from build123d import *

# Parameters (mm, degrees)
SKETCH_1_W               = 45
SKETCH_1_H               = 45
EXTRUDE_1_DEPTH          = 15
SKETCH_2_R               = 19
CUT_EXTRUDE_1_DEPTH      = 36.178118199
SKETCH_5_W               = 15
SKETCH_5_H               = 15
EXTRUDE_2_DEPTH          = 12
SKETCH_6_R               = 3
CUT_EXTRUDE_4_DEPTH      = 35
SKETCH_7_R               = 1.5
CUT_EXTRUDE_5_DEPTH      = 44.834917702
CUT_EXTRUDE_6_DEPTH      = 6
CUT_EXTRUDE_6_DEPTH_BACK = 6
SKETCH_9_R               = 4.25
CUT_EXTRUDE_7_DEPTH      = 12
CHAMFER_1_SIZE           = 2
CHAMFER_2_SIZE           = 1
CHAMFER_3_SIZE           = 1
CHAMFER_4_SIZE           = 1


# Some blends are built 0.0001 mm under size
with BuildPart() as part:
    # 草图1 → 凸台-拉伸1 (new body)
    with BuildSketch(Plane(origin=(0, 0, 0), x_dir=(1, 0, 0), z_dir=(0, 1, 0))):
        Rectangle(SKETCH_1_W, SKETCH_1_H)
    extrude(amount=EXTRUDE_1_DEPTH)

    # 草图2 → 切除-拉伸1 (cut, through all)
    with BuildSketch(Plane(origin=(0, 15, 0), x_dir=(1, 0, 0), z_dir=(0, 1, 0))):
        with Locations(Location((0, 0, 0), (0, 0, 270))):
            Circle(SKETCH_2_R)
    extrude(amount=-CUT_EXTRUDE_1_DEPTH, mode=Mode.SUBTRACT)

    # 草图5 → 凸台-拉伸2 (add)
    with BuildSketch(Plane(origin=(0, 0, -22.5), x_dir=(-1, 0, 0), z_dir=(0, 0, -1))):
        with Locations((14, 7.5)):
            Rectangle(SKETCH_5_W, SKETCH_5_H)
        with Locations((-14, 7.5)):
            Rectangle(SKETCH_5_W, SKETCH_5_H)
    extrude(amount=EXTRUDE_2_DEPTH)

    # 草图6 → 切除-拉伸4 (cut)
    with BuildSketch(Plane(origin=(0, 0, -34.5), x_dir=(-1, 0, 0), z_dir=(0, 0, -1))):
        with Locations((-14, 7.5)):
            Circle(SKETCH_6_R)
        with Locations((14, 7.5)):
            Circle(SKETCH_6_R)
    extrude(amount=-CUT_EXTRUDE_4_DEPTH, mode=Mode.SUBTRACT)

    # 草图7 → 切除-拉伸5 (cut, through all)
    with BuildSketch(Plane(origin=(0, 15, 0), x_dir=(1, 0, 0), z_dir=(0, 1, 0))):
        with Locations(Location((-19.5, 19.5, 0), (0, 0, 270))):
            Circle(SKETCH_7_R)
        with Locations(Location((19.5, 19.5, 0), (0, 0, 90))):
            Circle(SKETCH_7_R)
        with Locations(Location((19.5, -19.5, 0), (0, 0, 270))):
            Circle(SKETCH_7_R)
        with Locations(Location((-19.5, -19.5, 0), (0, 0, 90))):
            Circle(SKETCH_7_R)
    extrude(amount=-CUT_EXTRUDE_5_DEPTH, mode=Mode.SUBTRACT)

    # 草图8 → 切除-拉伸6 (cut, two sides: drawn at the far end of the back side and taken through both)
    with BuildSketch(Plane(origin=(0, 7.5, 0), x_dir=(-1, 0, 0), z_dir=(0, -1, 0)).offset(-CUT_EXTRUDE_6_DEPTH_BACK)):
        with BuildLine():
            Line((-8.874983497, 19.032463528), (-8.029746973, 17.219847954))
            ThreePointArc((-8.029746973, 17.219847954), (-15.073713466, 11.566467151), (-18.711347307, 3.299315376))
            Line((-18.711347307, 3.299315376), (-20.680962813, 3.646611731))
            ThreePointArc((-20.680962813, 3.646611731), (-16.660420146, 12.783990009), (-8.874983497, 19.032463528))
        make_face()
        with BuildLine():
            Line((20.680962813, 3.646611731), (18.711347307, 3.299315376))
            ThreePointArc((18.711347307, 3.299315376), (15.073713466, 11.566467151), (8.029746973, 17.219847954))
            Line((8.029746973, 17.219847954), (8.874983497, 19.032463528))
            ThreePointArc((8.874983497, 19.032463528), (16.660420146, 12.783990009), (20.680962813, 3.646611731))
        make_face()
    extrude(amount=CUT_EXTRUDE_6_DEPTH + CUT_EXTRUDE_6_DEPTH_BACK, mode=Mode.SUBTRACT)

    # 草图9 → 切除-拉伸7 (cut)
    with BuildSketch(Plane(origin=(0, 0, -34.5), x_dir=(-1, 0, 0), z_dir=(0, 0, -1))):
        with Locations((-14, 7.5)):
            Circle(SKETCH_9_R)
        with Locations((14, 7.5)):
            Circle(SKETCH_9_R)
    extrude(amount=-CUT_EXTRUDE_7_DEPTH, mode=Mode.SUBTRACT)

    # 倒角1
    # the kernel refuses this chamfer: 2 mm, written as the material it takes off along each edge
    with BuildSketch(Plane(origin=(-18.711347307, 1.5, -3.299315376), x_dir=(-0.11838916494267775, 0, 0.9929672731888879), z_dir=(0, 1, 0)), Plane(origin=(18.711347307, 13.5, -3.299315376), x_dir=(0.11838916494267755, 0, 0.9929672731888879), z_dir=(0, -1, 0))) as chamfer_1_piece_1:
        with BuildLine():
            Line((2.121782819, 0), (-CHAMFER_1_SIZE * 0.055836389964, -CHAMFER_1_SIZE * 0.998439931872))
            Line((-CHAMFER_1_SIZE * 0.055836389964, -CHAMFER_1_SIZE * 0.998439931872), (0, 0))
            ThreePointArc((0, 0), (1.090799435, -0.029617755), (2.121782819, 0))
        make_face()
    extrude(amount=12, mode=Mode.SUBTRACT)

    # 倒角2
    chamfer_2_edges = [part.edges().sort_by_distance(p)[0] for p in [
        (22.5, 7.5, 22.5),
        (-22.5, 7.5, 22.5),
        (-22.5, 7.5, -22.5),
        (22.5, 7.5, -22.5),
    ]]
    chamfer(chamfer_2_edges, length=CHAMFER_2_SIZE - 0.0001)  # a hair under: the kernel refuses the full size

    # 倒角3
    chamfer_3_edges = [part.edges().sort_by_distance(p)[0] for p in [
        (18.25, 7.5, -22.5),
        (-9.75, 7.5, -22.5),
    ]]
    chamfer(chamfer_3_edges, length=CHAMFER_3_SIZE)

    # 倒角4
    chamfer_4_edges = [part.edges().sort_by_distance(p)[0] for p in [
        (6.5, 7.5, -34.5),
        (14, 15, -34.5),
        (21.5, 7.5, -34.5),
        (14, 0, -34.5),
        (-21.5, 7.5, -34.5),
        (-14, 15, -34.5),
        (-6.5, 7.5, -34.5),
        (-14, 0, -34.5),
    ]]
    chamfer(chamfer_4_edges, length=CHAMFER_4_SIZE)


solid = part.part
Read the model definition and answer for the solid it produces. Units are mm, in the model's axes. A direction names the side the tool comes from. Coordinates: 2 decimals unless noted, no trailing zeros. Loops run counter-clockwise (first coordinate to the right, second up) from the corner with the lowest first, then second, coordinate; pieces in that order, holes last. Notation, with made-up numbers: (82.25, 73) -> (109.25, 73) arc R8 ccw to (109.25, 79) -> close; hole circle Ø1 at (79, 67). An arc over 180 degrees is marked (long way). Answer in a Markdown table with one row per item.
Item 1: Straight lines are drawn through the part: line 1 along X through (y, z) = (5, 19.5); line 2 along X through (y, z) = (8, -1); line 3 along X through (y, z) = (8, -19.5). For each, find the intervals that lie inside material, in ascending order. Write a range as [from, to].
Returned:
| item | result |
|---|---|
| line 1 | x = [-22.5, -21], [-18, 18], [21, 22.5] |
| line 2 | x = [-22.5, -18.97], [18.97, 22.5] |
| line 3 | x = [-22.5, -21], [-18, -16.96], [-11.04, 11.04], [16.96, 18], [21, 22.5] |
Item 2: For faces 4 (the cylindrical face through (17, 7.6, -18.6)), 5 (the flat face through (-16, 13.5, -11)), 6 (the flat face through (14, 12, -34.5)), 7 (the flat face through (-10, 15, -18)), 8 (the flat face through (0, 7, -22.5)), determine the directions among +Z, -Z, +X, -X, +Y, -Y from which every point of the face is accessible in a straight line to the end or side of a thin tool.
Returned:
| item | result |
|---|---|
| face 4 | -Z |
| face 5 | none |
| face 6 | -Z, +X, -X, +Y, -Y |
| face 7 | +Z, -Z, +X, -X, +Y |
| face 8 | -Z, +Y, -Y |
Item 3: A cutting plane is placed at A-A on z = -27. Determine the outline of the cut face in (x, y).
Returned:
| item | result |
|---|---|
| outline | (-21.5, 0) -> (-6.5, 0) -> (-6.5, 15) -> (-21.5, 15) -> close; (6.5, 0) -> (21.5, 0) -> (21.5, 15) -> (6.5, 15) -> close; hole circle Ø8.5 at (-14, 7.5); hole circle Ø8.5 at (14, 7.5) |
Item 4: A cutting plane is placed at D-D on z = 0. Determine the outline of the cut face in (x, y).
Returned:
| item | result |
|---|---|
| outline | (-22.5, 0) -> (-19, 0) -> (-19, 15) -> (-22.5, 15) -> close; (19, 0) -> (22.5, 0) -> (22.5, 15) -> (19, 15) -> close |
Item 5: A cutting plane is placed at B-B on y = 2.25. Give the number of separate pieces and of enclosed holes in the cut face, plus the area to 3 significant figures.
Returned:
| item | result |
|---|---|
| separate pieces | 1 |
| enclosed holes | 5 |
| area | 1,140 mm^2 |
Item 6: A cutting plane is placed at C-C on x = 0. Determine the outline of the cut face in (y, z), plus the area to 3 significant figures.
Returned:
| item | result |
|---|---|
| outline | (0, -22.5) -> (15, -22.5) -> (15, -19) -> (0, -19) -> close; (0, 19) -> (15, 19) -> (15, 22.5) -> (0, 22.5) -> close |
| area | 105 mm^2 |
Item 7: Each of these flat-tipped pins is pushed along its axis until it touches: P1, Ø2, axis at x = 14.5, y = 8.5, coming from the -Z side; P2, Ø5.5, axis at y = 10.5, z = -29, coming from the +X side; P3, Ø6.5, axis at x = -1.5, y = 4, coming from the -Z side; P4, Ø23, axis at x = 0, z = 0, coming from the -Y side. Where does it stop, or does it pass through?
Returned:
| item | result |
|---|---|
| P1 | stops at z = 10.99 |
| P2 | stops at x = 21.5 |
| P3 | stops at z = -22.5 |
| P4 | passes through |
Item 8: For a pull along X with two mould halves and no side action, classify faces 1 (the flat face through (-22.5, 7, 0)), 2 (the cylindrical face through (-18.49, 7.6, -20.61)), 3 (the flat face through (-14, 12, -34.5)) as released by +X, released by -X, zero draft, split by the parting line, or undercut.
Returned:
| item | result |
|---|---|
| face 1 | released by -X |
| face 2 | undercut |
| face 3 | zero draft |
